Input: part model. Units: mm. Frame: model coordinates. A direction names the side the tool comes from. Coordinates: 2 decimals unless noted, no trailing zeros. Order: outer loops, then holes, each group sorted by start corner. A loop starts at its lowest first (then second) coordinate and runs counter-clockwise, first axis right, second up.
from build123d import *

# Parameters (mm, degrees)
SALIENTE_EXTRUIR1_DEPTH = 11.8
CROQUIS2_R              = 2.3
SALIENTE_EXTRUIR2_DEPTH = 4
CROQUIS3_R              = 2.3
SALIENTE_EXTRUIR3_DEPTH = 7.2
CORTAR_EXTRUIR1_DEPTH   = 7.2
CROQUIS5_R              = 0.38741291
SALIENTE_EXTRUIR4_DEPTH = 1


with BuildPart() as part:
    # Croquis1 → Saliente-Extruir1 (new body)
    with BuildSketch(Plane.XY):
        Polygon((-10.840013315, -12.513302196), (11.659986685, -12.513302196), (11.659986685, 3.386697804), (16.359986685, 3.386697804), (16.359986685, 5.886697804), (11.659986685, 5.886697804), (11.659986685, 10.186697804), (-10.840013315, 10.186697804), (-10.840013315, 5.886697804), (-15.540013315, 5.886697804), (-15.540013315, 3.386697804), (-10.840013315, 3.386697804), align=None)
    extrude(amount=SALIENTE_EXTRUIR1_DEPTH)

    # Croquis2 → Saliente-Extruir2 (add)
    with BuildSketch(Plane(origin=(0, 10.186697804, 0), x_dir=(1, 0, 0), z_dir=(0, 1, 0))):
        with BuildLine():
            Line((1.359986685, -3.4), (0.404142371, -3.4))
            ThreePointArc((0.404142371, -3.4), (-10.840013315, -5.9), (0.404142371, -8.4))
            Line((0.404142371, -8.4), (1.359986685, -8.4))
            ThreePointArc((1.359986685, -8.4), (3.859986685, -5.9), (1.359986685, -3.4))
        make_face()
        with Locations(Location((-4.940013315, -5.9, 0), (0, 0, 270))):
            Circle(CROQUIS2_R, mode=Mode.SUBTRACT)
    extrude(amount=SALIENTE_EXTRUIR2_DEPTH)

    # Croquis3 → Saliente-Extruir3 (add)
    with BuildSketch(Plane(origin=(0, 10.186697804, 0), x_dir=(1, 0, 0), z_dir=(0, 1, 0))):
        with Locations(Location((-4.940013315, -5.9, 0), (0, 0, 270))):
            Circle(CROQUIS3_R)
    extrude(amount=SALIENTE_EXTRUIR3_DEPTH)

    # Croquis4 → Cortar-Extruir1 (cut)
    with BuildSketch(Plane(origin=(0, 5.886697804, 0), x_dir=(1, 0, 0), z_dir=(0, 1, 0))):
        with BuildLine():
            Line((16.359986685, -5.25), (16.359986685, -6.55))
            Line((16.359986685, -6.55), (14.819920893, -6.55))
            ThreePointArc((14.819920893, -6.55), (13.059986685, -5.9), (14.819920893, -5.25))
            Line((14.819920893, -5.25), (16.359986685, -5.25))
        make_face()
        with BuildLine():
            Line((-15.540013315, -6.55), (-15.540013315, -5.25))
            Line((-15.540013315, -5.25), (-13.999947523, -5.25))
            ThreePointArc((-13.999947523, -5.25), (-12.240013315, -5.9), (-13.999947523, -6.55))
            Line((-13.999947523, -6.55), (-15.540013315, -6.55))
        make_face()
    extrude(amount=-CORTAR_EXTRUIR1_DEPTH, mode=Mode.SUBTRACT)

    # Croquis5 → Saliente-Extruir4 (add)
    with BuildSketch(Plane(origin=(0, 17.386697804, 0), x_dir=(1, 0, 0), z_dir=(0, 1, 0))):
        with BuildLine():
            Line((3.522810247, -4.959091344), (-4.940013315, -3.6))
            Line((-4.940013315, -3.6), (-13.402836876, -4.959091344))
            ThreePointArc((-13.402836876, -4.959091344), (-14.343745532, -5.9), (-13.402836876, -6.840908656))
            Line((-13.402836876, -6.840908656), (-4.940013315, -8.2))
            Line((-4.940013315, -8.2), (3.522810247, -6.840908656))
            ThreePointArc((3.522810247, -6.840908656), (4.463718903, -5.9), (3.522810247, -4.959091344))
        make_face()
        with Locations(Location((3.522810247, -5.9, 0), (0, 0, 270))):
            Circle(CROQUIS5_R, mode=Mode.SUBTRACT)
        with Locations(Location((2.022810247, -5.9, 0), (0, 0, 270))):
            Circle(CROQUIS5_R, mode=Mode.SUBTRACT)
        with Locations(Location((0.522810247, -5.9, 0), (0, 0, 270))):
            Circle(CROQUIS5_R, mode=Mode.SUBTRACT)
        with Locations(Location((-0.977189753, -5.9, 0), (0, 0, 270))):
            Circle(CROQUIS5_R, mode=Mode.SUBTRACT)
        with Locations(Location((-13.402836876, -5.9, 0), (0, 0, 270))):
            Circle(CROQUIS5_R, mode=Mode.SUBTRACT)
        with Locations(Location((-11.902836876, -5.9, 0), (0, 0, 270))):
            Circle(CROQUIS5_R, mode=Mode.SUBTRACT)
        with Locations(Location((-10.402836876, -5.9, 0), (0, 0, 270))):
            Circle(CROQUIS5_R, mode=Mode.SUBTRACT)
        with Locations(Location((-8.902836876, -5.9, 0), (0, 0, 270))):
            Circle(CROQUIS5_R, mode=Mode.SUBTRACT)
    extrude(amount=-SALIENTE_EXTRUIR4_DEPTH)


solid = part.part
Item 1: Access query for faces 1 (the face through (-0.4, 16.89, 7.47)), 2 (the face through (-10.84, 8, 6)), 3 (the face through (12.9, 3.387, 5.8)). Directions: +Z, -Z, +X, -X, +Y, -Y. A direction counts if a zero-diameter tool reaches every point of the face in a straight line with its end or side. Return the directions, or none.
Response values:
face 1: +Z, +X, +Y
face 2: +Z, -Z, -X
face 3: +Z, -Z, +X, -Y
Item 2: Cut plane A-A on z = 10.75. Return loops of the section in (x, y), then the cut area to 3 significant figures.
Response values:
outline: (-15.54, 3.39) - (-10.84, 3.39) - (-10.84, -12.51) - (11.66, -12.51) - (11.66, 3.39) - (16.36, 3.39) - (16.36, 5.89) - (11.66, 5.89) - (11.66, 10.19) - (-1.58, 10.19) - (-1.58, 14.19) - (-8.3, 14.19) - (-8.3, 10.19) - (-10.84, 10.19) - (-10.84, 5.89) - (-15.54, 5.89) - close
area: 561 mm2
Item 3: Pin query (flat end, axial travel): pin 1 Ø1.8 at (x, z) = (-8.5, 3) entering from +Y; pin 2 Ø1.4 at (x, z) = (14.5, 4) entering from -Y; pin 3 Ø0.8 at (x, y) = (1, 12.5) entering from +Z. Return the tip coordinate at first contact, or that it passes through.
Response values:
pin 1: stops at y = 14.19
pin 2: stops at y = 3.39
pin 3: stops at z = 8.4
Item 4: Cut plane D-D on z = 1.25. Return loops of the section in (x, y).
Response values:
outline: (-15.54, 3.39) - (-10.84, 3.39) - (-10.84, -12.51) - (11.66, -12.51) - (11.66, 3.39) - (16.36, 3.39) - (16.36, 5.89) - (11.66, 5.89) - (11.66, 10.19) - (-1.31, 10.19) - (-1.31, 14.19) - (-8.57, 14.19) - (-8.57, 10.19) - (-10.84, 10.19) - (-10.84, 5.89) - (-15.54, 5.89) - close
Item 5: Draft query along Z for faces 4 (the face through (1, 12, 3.4)), 5 (the face through (-15, 5, 6.55)), 6 (the face through (16, 5, 6.55)), 7 (the face through (0, -1, 11.8)). Return one class per face: pulls with the +Z half, pulls with the -Z half, needs draft (parallel to the pull), parting line crosses it, or undercut.
Response values:
face 4: pulls with the -Z half
face 5: undercut
face 6: undercut
face 7: pulls with the +Z half
Item 6: Cut plane C-C on y = 15.25. Return loops of the section in (x, z).
Response values:
outline: circle Ø4.6 at (-4.94, 5.9)
Item 7: Ray query, probe 1 along Y at (x, z) = (-1, 6.5); probe 2 along Y at (x, z) = (-11, 4.75); probe 3 along Y at (x, z) = (-10, 2.5). Return the intervals inside material, ascending.
Response values:
probe 1: y = -12.51 to 14.19, 16.39 to 17.39
probe 2: y = 3.39 to 5.89, 16.39 to 17.39
probe 3: y = -12.51 to 10.19
Item 8: Cut plane B-B on x = 6.5. Return loops of the section in (y, z), then the cut area to 3 significant figures.
Response values:
outline: (-12.51, 0) - (10.19, 0) - (10.19, 11.8) - (-12.51, 11.8) - close
area: 268 mm2
